from build123d import *

# Parameters (mm, degrees)
SKETCH1_W           = 105
SKETCH1_H           = 12.3
BOSS_EXTRUDE1_DEPTH = 5
SKETCH2_W           = 5
SKETCH2_H           = 5
BOSS_EXTRUDE2_DEPTH = 5
SKETCH3_W           = 73
SKETCH3_H           = 5
CUT_EXTRUDE1_DEPTH  = 17
SKETCH4_W           = 5
SKETCH4_H           = 5
BOSS_EXTRUDE3_DEPTH = 5
SKETCH5_W           = 5
SKETCH5_H           = 15
BOSS_EXTRUDE4_DEPTH = 5


with BuildPart() as part:
    # Sketch1 → Boss-Extrude1 (new body)
    with BuildSketch(Plane.XY):
        Rectangle(SKETCH1_W, SKETCH1_H)
    extrude(amount=BOSS_EXTRUDE1_DEPTH)

    # Sketch2 → Boss-Extrude2 (add)
    with BuildSketch(Plane.XZ.offset(6.15)):
        with Locations((50, 2.5)):
            Rectangle(SKETCH2_W, SKETCH2_H)
    extrude(amount=BOSS_EXTRUDE2_DEPTH)

    # Mirror1: part across plane


with BuildPart() as part_1:
    add(part.part)
    add(part.part.mirror(Plane(origin=(-52.5, 6.15, 5), x_dir=(0, 0, 1), z_dir=(0, -1, 0))))

    # Sketch3 → Cut-Extrude1 (cut)
    with BuildSketch(Plane(origin=(0, 18.45, 0), x_dir=(1, 0, 0), z_dir=(0, 1, 0))):
        with Locations((6.5, -2.5)):
            Rectangle(SKETCH3_W, SKETCH3_H)
    extrude(amount=-CUT_EXTRUDE1_DEPTH, mode=Mode.SUBTRACT)

    # Sketch4 → Boss-Extrude3 (add)
    with BuildSketch(Plane.XZ.offset(6.15)):
        with Locations((0, 2.5)):
            Rectangle(SKETCH4_W, SKETCH4_H)
        with Locations((-50, 2.5)):
            Rectangle(SKETCH4_W, SKETCH4_H)
    extrude(amount=BOSS_EXTRUDE3_DEPTH)

    # Sketch5 → Boss-Extrude4 (add)
    with BuildSketch(Plane.ZY.offset(52.5)):
        with Locations((2.5, 6.15)):
            Rectangle(SKETCH5_W, SKETCH5_H)
    boss_extrude4 = extrude(amount=BOSS_EXTRUDE4_DEPTH)

    # Mirror2: Boss-Extrude4 across plane
    add(boss_extrude4.mirror(Plane(origin=(0, 0, 0), x_dir=(0, 0, 1), z_dir=(1, 0, 0))))


solid = part_1.part
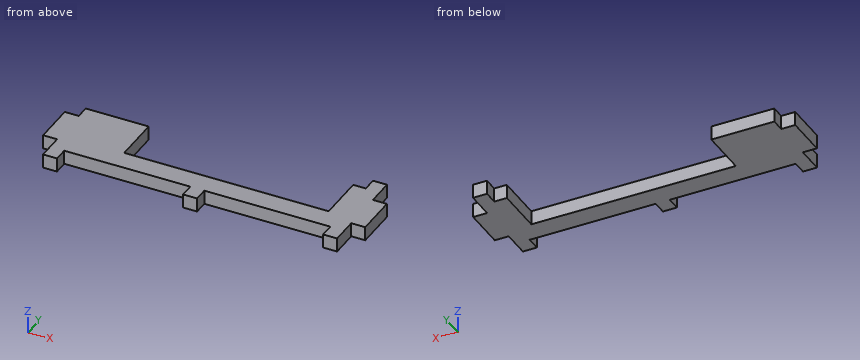
Verification items for the finished model (mm, model axes). Round coordinates to 2 decimals unless told otherwise and drop trailing zeros. Write each loop counter-clockwise with the first axis right and the second up, starting at its lowest first coordinate (ties: lowest second). Pieces come first, ordered by that corner, then holes.
(1) Section check D-D (y = 15.5). Enter the section's corners in (x, z).
Returned:
outline: (-52.5, 0) - (-30, 0) - (-30, 5) - (-52.5, 5) - close; (43, 0) - (52.5, 0) - (52.5, 5) - (43, 5) - close
(2) Section check A-A (y = 4.5). Enter the section's corners in (x, z), plus the area to 3 significant figures.
Returned:
outline: (-57.5, 0) - (-30, 0) - (-30, 5) - (-57.5, 5) - close; (43, 0) - (57.5, 0) - (57.5, 5) - (43, 5) - close
area: 210 mm2
(3) Depth check by flat-ended pin: pin 1 Ø1 at (x, z) = (45.5, 3) entering from +Y; pin 2 Ø2.5 at (x, z) = (26, 2) entering from -Y; pin 3 Ø1.5 at (y, z) = (-3, 1) entering from -X; pin 4 Ø2 at (y, z) = (-1.5, 2.5) entering from -X. Enter the tip coordinate at first touch or a pass-through.
Returned:
pin 1: stops at y = 18.45
pin 2: stops at y = -6.15
pin 3: stops at x = -52.5
pin 4: stops at x = -57.5
(4) Material ranges on line 1 (X direction, y = -9, z = 2.8); line 2 (X direction, y = 7, z = 4.75); line 3 (Y direction, x = -12, z = 3.5), recorded low to high.
Returned:
line 1: x = -52.5 to -47.5, -2.5 to 2.5, 47.5 to 52.5
line 2: x = -57.5 to -30, 43 to 57.5
line 3: y = -6.15 to 1.45
(5) Section check B-B (z = 1). Enter the section's corners in (x, y).
Returned:
outline: (-57.5, -1.35) - (-52.5, -1.35) - (-52.5, -11.15) - (-47.5, -11.15) - (-47.5, -6.15) - (-2.5, -6.15) - (-2.5, -11.15) - (2.5, -11.15) - (2.5, -6.15) - (47.5, -6.15) - (47.5, -11.15) - (52.5, -11.15) - (52.5, -1.35) - (57.5, -1.35) - (57.5, 13.65) - (52.5, 13.65) - (52.5, 23.45) - (47.5, 23.45) - (47.5, 18.45) - (43, 18.45) - (43, 1.45) - (-30, 1.45) - (-30, 18.45) - (-52.5, 18.45) - (-52.5, 13.65) - (-57.5, 13.65) - close
(6) Section check C-C (y = -8). Enter the section's corners in (x, z).
Returned:
outline: (-52.5, 0) - (-47.5, 0) - (-47.5, 5) - (-52.5, 5) - close; (-2.5, 0) - (2.5, 0) - (2.5, 5) - (-2.5, 5) - close; (47.5, 0) - (52.5, 0) - (52.5, 5) - (47.5, 5) - close
